Geometry: final body of the model. Coordinates: model frame, mm. A direction names the side the tool comes from. Give positions to 0.01 mm unless a question says otherwise; leave off trailing zeros. Loops run counter-clockwise (first coordinate to the right, second up) from the corner with the lowest first, then second, coordinate; pieces in that order, holes last. Notation, with made-up numbers: (88.5, 13) - (145.5, 13) arc R20 cw to (145.5, 36) - close; hole circle Ø8 at (34.25, 1.25). An arc over 180 degrees is marked (long way). Use CSV: the item, a comma, the result in double quotes. Start each with the question number.
```python
from build123d import *

# Parameters (mm, degrees)
F1_DEPTH  = 25.4
F2_R      = 1.5748
F3_DEPTH  = 12.7
F4_R      = 1.5748
F5_DEPTH  = 12.7
F6_R      = 1.5748
F7_DEPTH  = 12.7
F8_R      = 1.5748
F9_DEPTH  = 12.7
F10_R     = 1.5748
F11_DEPTH = 12.7


with BuildPart() as f1:
    # F0 (on Front) → F1 (new body)
    with BuildSketch(Plane.XZ):
        Polygon((4.777168, 54.35802), (-33.003355, -11.521775), (43.069369, -11.521775), align=None)
    extrude(amount=F1_DEPTH)

    # F2 (on face) → F3 (cut)
    with BuildSketch(Plane.XZ.offset(25.4)):
        with Locations((-21.482399, -5.251253)):
            Circle(F2_R)
        with Locations((-7.924618, -5.251253)):
            Circle(F2_R)
        with Locations((5.442207, -5.251253)):
            Circle(F2_R)
        with Locations((18.999988, -5.251253)):
            Circle(F2_R)
        with Locations((32.557771, -5.251253)):
            Circle(F2_R)
    extrude(amount=-F3_DEPTH, mode=Mode.SUBTRACT)

    # F4 (on face) → F5 (cut)
    with BuildSketch(Plane.XZ.offset(25.4)):
        with Locations((-13.462303, 9.070346)):
            Circle(F4_R)
        with Locations((0, 9.070346)):
            Circle(F4_R)
        with Locations((11.934667, 9.070346)):
            Circle(F4_R)
        with Locations((24.728628, 9.070346)):
            Circle(F4_R)
    extrude(amount=-F5_DEPTH, mode=Mode.SUBTRACT)

    # F6 (on face) → F7 (cut)
    with BuildSketch(Plane.XZ.offset(25.4)):
        with Locations((-6.015072, 23.010036)):
            Circle(F6_R)
        with Locations((4.777168, 23.010036)):
            Circle(F6_R)
        with Locations((16.51758, 23.010036)):
            Circle(F6_R)
    extrude(amount=-F7_DEPTH, mode=Mode.SUBTRACT)

    # F8 (on face) → F9 (cut)
    with BuildSketch(Plane.XZ.offset(25.4)):
        with Locations((0, 35.613045)):
            Circle(F8_R)
        with Locations((10.407028, 35.613045)):
            Circle(F8_R)
    extrude(amount=-F9_DEPTH, mode=Mode.SUBTRACT)

    # F10 (on face) → F11 (cut)
    with BuildSketch(Plane.XZ.offset(25.4)):
        with Locations((4.869344, 46.879366)):
            Circle(F10_R)
    extrude(amount=-F11_DEPTH, mode=Mode.SUBTRACT)


solid = f1.part
```
Item 1: Section B-B (y = -10). Output: boundary loops of the cut face in (x, z).
Item 2: Pin query (flat end, axial travel): pin 1 Ø1.9 at (x, z) = (-13.46, 9.07) entering from -Y; pin 2 Ø5 at (y, z) = (-16, -4) entering from -X; pin 3 Ø2.5 at (x, z) = (16.52, 23.01) entering from +Y; pin 4 Ø4 at (x, y) = (-8, -9) entering from +Z. Return the tip coordinate at first contact, or that it passes through.
Item 3: Section D-D (z = 33). Output: boundary loops of the cut face in (x, y).
Item 4: Section A-A (y = -23.25). Give the number of separate pieces and of enclosed holes in the cut face, plus the area to 3 significant figures.
Item 5: Reachability of faces 1 (the flat face through (5, -25.4, 7)), 2 (the flat face through (-13, -12.7, 9)) from +Z, -Z, +X, -X, +Y, -Y: full face, straight path, thin tool, end or side. Return the list, or none.
Item 6: Section C-C (x = 0). Output: boundary loops of the cut face in (y, z).
Item 7: Ray query, probe 1 along Z at (x, y) = (11, -15.75); probe 2 along X at (y, z) = (-22.25, 37); probe 3 along Z at (x, y) = (19, -22). Return the intervals inside material, ascending.
Outcome:
1,outline,"(-33, -11.52) - (43.07, -11.52) - (4.78, 54.36) - close"
2,pin 1,"stops at y = -12.7"
2,pin 2,"stops at x = -30.12"
2,pin 3,"stops at y = 0"
2,pin 4,"stops at z = 35.57"
3,outline,"(-7.47, -25.4) - (17.19, -25.4) - (17.19, 0) - (-7.47, 0) - close"
4,separate pieces,"1"
4,enclosed holes,"15"
4,area,"2,390 mm2"
5,face 1,"+Z, -Z, +X, -X, -Y"
5,face 2,"-Y"
6,outline,"(-25.4, -11.52) - (0, -11.52) - (0, 46.03) - (-25.4, 46.03) - (-25.4, 37.19) - (-12.7, 37.19) - (-12.7, 34.04) - (-25.4, 34.04) - (-25.4, 10.65) - (-12.7, 10.65) - (-12.7, 7.5) - (-25.4, 7.5) - close"
7,probe 1,"z = -11.52 to 7.8, 10.34 to 34.15, 37.07 to 43.65"
7,probe 2,"x = -5.18 to -0.75, 0.75 to 9.66, 11.15 to 14.87"
7,probe 3,"z = -11.52 to -6.83, -3.68 to 29.89"
